Part model, mm, in its own coordinate system. A direction names the side the tool comes from. Round coordinates to 2 decimals unless told otherwise and drop trailing zeros. Write each loop counter-clockwise with the first axis right and the second up, starting at its lowest first coordinate (ties: lowest second). Pieces come first, ordered by that corner, then holes. Notation, with made-up numbers: M 7,-37.5 L 33,-37.5 A25 cw 33,-4.5 Z; hole C 82.25,82 d11. An arc over 180 degrees is marked long. Answer as a JSON object with one key per item and string values. Group by question number.
1. Band-saw the part on C-C, the plane z = 92.5. Write the cut outline in (x, y).
2. Drill centre lines: line 1 (Z direction, x = -89, y = 93.5); line 2 (Y direction, x = -71.5, z = 92.5); line 3 (X direction, y = 87.5, z = 95.25). Where is each one in solid material? Low to high. Write a range as from..to.
3. Drop a flat-ended pin along its axis: pin 1 (2 mm diameter, centred on y = 95, z = 93, fed in from -X). Give the stop position or say it passes through.
4. Two-plate mould, pull along X, no slides. Class faces 1 (the face through (-89, 94, 98.051)), 2 (the face through (-113.6, 80.36, 96.02)), 3 (the face through (-73.83, 96.48, 92.08)): +X half, -X half, draft (parallel to the pull), parting line (faces both ways), or undercut.
5. Band-saw the part on A-A, the plane y = 88.25. Write the cut outline in (x, z).
6. Band-saw the part on B-B, the plane x = -73.5. Write the cut outline in (y, z).
7. Band-saw the part on D-D, the plane y = 94. Write the cut outline in (x, z), plus the area to 3 significant figures.
8. Which spindle directions (+Z, -Z, +X, -X, +Y, -Y) get a long thin tool onto all of the face, cutting with end or side? Do faces 4 (the face through (-114.5, 94, 96)), 5 (the face through (-101.115, 94.751, 92.079)). Say none if no direction does.
Solid Edge part; units mm, degrees
sketch "Sketch1" plane through (0, 0, 98.0511) normal (0, 0, 1) x (1, 0, 0)
  line L0 (-114.5, 79.5) -> (-62.5, 79.5)
  line L1 (-62.5, 79.5) -> (-62.5, 108.5)
  line L2 (-114.5, 108.5) -> (-62.5, 108.5)
  line L3 (-114.5, 108.5) -> (-114.5, 79.5)
extrude "Protrusion1" add sketch "Sketch1" against normal blind 4
fillet "Round_3" radius 3 2 edges at (-114.5, 79.5, 96.0511) (-114.5, 108.5, 96.0511)
chamfer "Chamfer_2" distance 1.5 angle 45 1 edges at (-62.5, 94, 94.0511)
fillet "Round_4" radius 3 2 edges at (-62.5, 79.5, 96.8011) (-62.5, 108.5, 96.8011)
sketch "Sketch2" plane through (-89.25, 94, 94.0511) normal (0, 0, -1) x (1, 0, 0)
  circle A0 centre (-14.25, 0) radius 2.5
  circle A1 centre (15.75, 0) radius 2.5
extrude "ExtrudedProtrusion_8" add sketch "Sketch2" along normal blind 4
Worked answers:
{
 "1": {"outline": "C -103.5,94 d5; C -73.5,94 d5"},
 "2": {"line 1": "z = 94.05..98.05", "line 2": "y = 92.5..95.5", "line 3": "x = -114.5..-62.8"},
 "3": {"pin 1": "stops at x = -106"},
 "4": {"face 1": "draft", "face 2": "-X half", "face 3": "undercut"},
 "5": {"outline": "M -114.5,94.05 L -64,94.05 L -62.5,95.55 L -62.5,98.05 L -114.5,98.05 Z"},
 "6": {"outline": "M 79.5,94.05 L 91.5,94.05 L 91.5,90.05 L 96.5,90.05 L 96.5,94.05 L 108.5,94.05 L 108.5,98.05 L 79.5,98.05 Z"},
 "7": {"outline": "M -114.5,94.05 L -106,94.05 L -106,90.05 L -101,90.05 L -101,94.05 L -76,94.05 L -76,90.05 L -71,90.05 L -71,94.05 L -64,94.05 L -62.5,95.55 L -62.5,98.05 L -114.5,98.05 Z", "area": "247 mm^2"},
 "8": {"face 4": "+Z, -Z, -X, +Y, -Y", "face 5": "-Z"}
}
